Input: part model. Units: mm. Frame: model coordinates. Face numbers are marked on the shaded views. A direction names the side the tool comes from. Coordinates: 2 decimals unless noted, no trailing zeros. Order: outer loops, then holes, each group sorted by start corner. A loop starts at its lowest first (then second) coordinate and runs counter-clockwise, first axis right, second up. Notation, with made-up numbers: (81.5, 78.5) - (121.5, 78.5) arc R30 ccw to (121.5, 106.5) - close; hole circle Ø7 at (-18, 89.5). An arc over 180 degrees is marked (long way). Use a Markdown table: item, result. Add a question column.
from build123d import *

# Parameters (mm, degrees)
PAD_DEPTH       = 8.5
SKETCH001_W     = 16
SKETCH001_H     = 13
POCKET_DEPTH    = 16
POCKET001_DEPTH = 5
POCKET002_DEPTH = 5
SKETCH004_W     = 2
SKETCH004_H     = 4
PAD001_DEPTH    = 1
SKETCH005_W     = 2
SKETCH005_H     = 4
PAD002_DEPTH    = 1
CHAMFER_SIZE    = 0.25
CHAMFER001_SIZE = 0.25
CHAMFER002_SIZE = 0.25


with BuildPart() as part:
    # Sketch → Pad (new body, symmetric)
    with BuildSketch(Plane.XZ):
        Polygon((0, 0), (20, 0), (20, 4), (4, 20), (0, 20), align=None)
    extrude(amount=PAD_DEPTH, both=True)

    # Sketch001 (on Face4 of Pad) → Pocket (cut)
    with BuildSketch(Plane(origin=(0, 0, 20), x_dir=(-1, 0, 0), z_dir=(0, 0, 1))):
        with Locations((-12, 0)):
            Rectangle(SKETCH001_W, SKETCH001_H)
    extrude(amount=-POCKET_DEPTH, mode=Mode.SUBTRACT)

    # Sketch002 (on Face2 of Pocket) → Pocket001 (cut)
    with BuildSketch(Plane(origin=(0, 0, 0), x_dir=(0, 0, -1), z_dir=(-1, 0, 0))):
        with BuildLine():
            ThreePointArc((-13, 3), (-16, 0), (-13, -3))
            Line((-13, -3), (-10, -3))
            ThreePointArc((-10, -3), (-7, 0), (-10, 3))
            Line((-13, 3), (-10, 3))
        make_face()
    extrude(amount=-POCKET001_DEPTH, mode=Mode.SUBTRACT)

    # Sketch003 (on Face1 of Pocket001) → Pocket002 (cut)
    with BuildSketch(Plane(origin=(0, 0, 0), x_dir=(1, 0, 0), z_dir=(0, 0, -1))):
        with BuildLine():
            ThreePointArc((10, 3), (7, 0), (10, -3))
            Line((10, -3), (13, -3))
            ThreePointArc((13, -3), (16, 0), (13, 3))
            Line((10, 3), (13, 3))
        make_face()
    extrude(amount=-POCKET002_DEPTH, mode=Mode.SUBTRACT)

    # Sketch004 (on Face1 of Pocket002) → Pad001 (join)
    with BuildSketch(Plane(origin=(0, 0, 0), x_dir=(1, 0, 0), z_dir=(0, 0, -1))):
        with Locations((3.5, 0)):
            Rectangle(SKETCH004_W, SKETCH004_H)
        with Locations((17.5, 0)):
            Rectangle(SKETCH004_W, SKETCH004_H)
    extrude(amount=PAD001_DEPTH)

    # Sketch005 (on Face2 of Pad001) → Pad002 (join)
    with BuildSketch(Plane(origin=(0, 0, 0), x_dir=(0, 0, -1), z_dir=(-1, 0, 0))):
        with Locations((-17.5, 0)):
            Rectangle(SKETCH005_W, SKETCH005_H)
        with Locations((-3.5, 0)):
            Rectangle(SKETCH005_W, SKETCH005_H)
    extrude(amount=PAD002_DEPTH)

    # Chamfer
    chamfer_edges = [part.edges().sort_by_distance(p)[0] for p in [
        (2, -8.5, 20),
        (0, -8.5, 10),
        (10, -8.5, 0),
        (0, 0, 0),
        (10, 8.5, 0),
        (0, 8.5, 10),
        (20, 0, 0),
        (20, 8.5, 2),
        (20, -8.5, 2),
        (16, 0, 4),
        (16, 0, 0),
        (0, 0, 7),
        (0, 0, 20),
        (2, 8.5, 20),
        (12, -8.5, 12),
        (12, 8.5, 12),
        (20, 0, 4),
        (4, 0, 16),
        (4, 0, 20),
    ]]
    chamfer(chamfer_edges, length=CHAMFER_SIZE)

    # Chamfer001
    chamfer001_edges = [part.edges().sort_by_distance(p)[0] for p in [
        (12, -6.5, 12),
    ]]
    chamfer(chamfer001_edges, length=CHAMFER001_SIZE)

    # Chamfer002
    chamfer002_edges = [part.edges().sort_by_distance(p)[0] for p in [
        (12, 6.5, 12),
    ]]
    chamfer(chamfer002_edges, length=CHAMFER002_SIZE)


solid = part.part
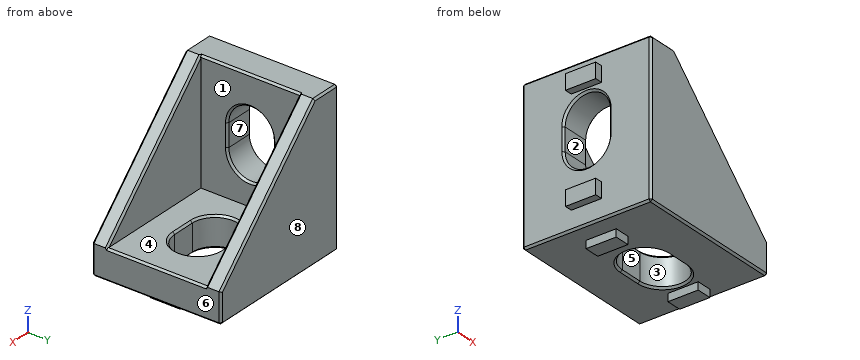
1) Reachability of the marked faces 4, 5, 6, 7 and 8 from +Z, -Z, +X, -X, +Y, -Y: full face, straight path, thin tool, end or side. Return the list, or none.
2) Contact query for flat-ended pins moving along their axis: P1, Ø5, axis at y = -2.5, z = 8, coming from the -X side; P2, Ø1.1, axis at y = -0.5, z = -0.5, coming from the -X side; P3, Ø2, axis at y = 5, z = 9.5, coming from the +X side; P4, Ø8, axis at x = 15, z = 15.5, coming from the +Y side. Output: stop coordinate, or through.
3) Cut plane A-A (y = -5.75). Return the cut outline in (x, z), and give its area (3 significant figures).
4) Pull-direction query (X, two-part tool) for the marked faces 1, 2 and 3; classes: pulls with the +X half, pulls with the -X half, needs draft (parallel to the pull), parting line crosses it, or undercut.
5) Cut plane D-D (y = 0). State how many separate pieces and enclosed holes the cut face has, and give its area (3 significant figures).
6) Cut plane C-C (x = 17). Return the cut outline in (y, z).
7) Cut plane B-B (z = 11). Return the cut outline in (x, y), and give its area (3 significant figures).
8) Material intervals for L1, parallel to Y at x = 4.5, z = 12.75; L2, parallel to Y at x = 2.75, z = 10; L3, parallel to X at y = -4.5, z = 0.5, sorted ascending.
Computed:
| question | item | result |
|---|---|---|
| 1 | face 4 | +Z, +X |
| 1 | face 5 | +Z, -Z |
| 1 | face 6 | +Z, -Z, +X, +Y, -Y |
| 1 | face 7 | +X, -X |
| 1 | face 8 | +Z, -Z, +X, -X, +Y |
| 2 | P1 | stops at x = 0 |
| 2 | P2 | stops at x = 0.2 |
| 2 | P3 | stops at x = 4 |
| 2 | P4 | passes through |
| 3 | outline | (0, 0.25) - (0.25, 0) - (19.75, 0) - (20, 0.25) - (20, 3.75) - (19.75, 4) - (4, 4) - (4, 19.75) - (3.75, 20) - (0.25, 20) - (0, 19.75) - close |
| 3 | area | 144 mm2 |
| 4 | face 1 | pulls with the +X half |
| 4 | face 2 | needs draft |
| 4 | face 3 | undercut |
| 5 | separate pieces | 3 |
| 5 | enclosed holes | 0 |
| 5 | area | 79.6 mm2 |
| 6 | outline | (-8.5, 0.25) - (-8.25, 0) - (-2, 0) - (-2, -1) - (2, -1) - (2, 0) - (8.25, 0) - (8.5, 0.25) - (8.5, 6.65) - (8.25, 7) - (6.75, 7) - (6.5, 6.65) - (6.5, 4) - (-6.5, 4) - (-6.5, 6.65) - (-6.75, 7) - (-8.25, 7) - (-8.5, 6.65) - close |
| 7 | outline | (0, -8.25) - (0.25, -8.5) - (12.65, -8.5) - (13, -8.25) - (13, -6.75) - (12.65, -6.5) - (4, -6.5) - (4, -3.25) - (3.75, -3) - (0.25, -3) - (0, -3.25) - close; (0, 3.25) - (0.25, 3) - (3.75, 3) - (4, 3.25) - (4, 6.5) - (12.65, 6.5) - (13, 6.75) - (13, 8.25) - (12.65, 8.5) - (0.25, 8.5) - (0, 8.25) - close |
| 7 | area | 79.6 mm2 |
| 8 | L1 | y = -8.5 to -6.5, 6.5 to 8.5 |
| 8 | L2 | y = -8.5 to -3, 3 to 8.5 |
| 8 | L3 | x = 0 to 20 |
